The listing builds one solid part. Answer for the finished solid, in the listing's coordinates (mm). A direction names the side the tool comes from. Give positions to 0.01 mm unless a question says otherwise; leave off trailing zeros. Write each loop counter-clockwise with the first axis right and the second up, starting at its lowest first coordinate (ties: lowest second). Pieces come first, ordered by that corner, then holes. Notation, with made-up numbers: (-22.75, 39) - (20.25, 39) arc R16 ccw to (20.25, 54) - close; hole circle Ø11 at (32, 9). An arc over 180 degrees is marked (long way). Answer as CSV lines item,"result". Start each with the question number.
(1) Find section C-C (y = -13.5). Write down the section's boundary in (x, z).
(2) Straight lines are drawn through the part: probe 1 along X at (y, z) = (-4.5, 25); probe 2 along Z at (x, y) = (8.5, -11); probe 3 along Y at (x, z) = (-34, -5). For each, find the intervals that lie inside material, in ascending order.
(3) Each of these flat-tipped pins is pushed along its axis until it touches: pin 1 Ø12 at (x, y) = (2, -28.5) entering from -Z; pin 2 Ø9 at (y, z) = (-27.5, 2.5) entering from +X; pin 3 Ø9 at (x, y) = (-1.5, -30.5) entering from +Z. Where does it stop, or does it pass through?
(4) Find section B-B (z = 32). Write down the section's boundary in (x, y).
(5) Find section D-D (x = 18.5). Write down the section's boundary in (y, z), then the cut area to 3 significant figures.
(6) Find section A-A (x = -35). Write down the section's boundary in (y, z).
(7) For faces 1 (the face through (-7.337, -2.702, 23.943)), 2 (the face through (7.287, -33.942, 7.248)), 3 (the face through (-7.248, -33.942, -7.287)), 4 (the face through (8.05, -10, 24)), determine the directions among +Z, -Z, +X, -X, +Y, -Y from which every point of the face is accessible in a straight line to the end or side of a thin tool.
from build123d import *

# Parameters (mm, degrees)
F0_W     = 16
F0_H     = 16
F1_DEPTH = 50
F0_W_2   = 20
F0_H_2   = 20
F2_DEPTH = 20
F3_W     = 16
F3_H     = 16
F4_DEPTH = 40
F5_W     = 16
F5_H     = 16
F6_DEPTH = 40
F7_W     = 16.1
F7_H     = 16.1
F8_DEPTH = 40
F9_R     = 2.5


with BuildPart() as f1:
    # F0 (on Front) → F1 (new body)
    with BuildSketch(Plane.XZ):
        Rectangle(F0_W, F0_H)
    extrude(amount=F1_DEPTH)

    # F0 (on Front) → F2 (join)
    with BuildSketch(Plane.XZ):
        Rectangle(F0_W_2, F0_H_2)
        Rectangle(F0_W, F0_H, mode=Mode.SUBTRACT)
    extrude(amount=F2_DEPTH)

    # F3 (on Right) → F4 (join)
    with BuildSketch(Plane.YZ):
        with Locations((-9.85, 0)):
            Rectangle(F3_W, F3_H)
    extrude(amount=F4_DEPTH)

    # F5 (on Right) → F6 (join)
    with BuildSketch(Plane.YZ):
        with Locations((-10, 0)):
            Rectangle(F5_W, F5_H)
    extrude(amount=-F6_DEPTH)

    # F7 (on Top) → F8 (join)
    with BuildSketch(Plane.XY):
        with Locations((0, -10)):
            Rectangle(F7_W, F7_H)
    extrude(amount=F8_DEPTH)

    # F9
    f9_edges = [f1.edges().sort_by_distance(p)[0] for p in [
        (0, 0, -10),
        (-25, -2, -8),
        (-25, -18, -8),
        (-25, -2, 8),
        (-25, -18, 8),
        (-40, -10, -8),
        (-40, -2, 0),
        (-40, -10, 8),
        (-40, -18, 0),
        (-8.05, -18.05, 25),
        (0, -18.05, 40),
        (-8.05, -10, 40),
        (8.05, -10, 40),
        (0, -1.95, 40),
        (-8.05, -1.95, 25),
        (8.05, -1.95, 25),
        (8.05, -18.05, 25),
        (-8, -35, 8),
        (0, -50, 8),
        (8, -35, 8),
        (-8, -50, 0),
        (0, -50, -8),
        (8, -50, 0),
        (25, -17.85, 8),
        (25, -17.85, -8),
        (40, -9.85, -8),
        (40, -1.85, 0),
        (40, -9.85, 8),
        (40, -17.85, 0),
        (8, -35, -8),
        (-8, -35, -8),
        (25, -1.85, -8),
    ]]
    fillet(f9_edges, radius=F9_R)


solid = f1.part
Result set:
1,outline,"(-40, -5.5) arc R2.5 ccw to (-37.5, -8) - (-10, -8) - (-10, -10) - (10, -10) - (10, -8) - (37.5, -8) arc R2.5 ccw to (40, -5.5) - (40, 5.5) arc R2.5 ccw to (37.5, 8) - (10, 8) - (10, 10) - (8.05, 10) - (8.05, 37.5) arc R2.5 ccw to (5.55, 40) - (-5.55, 40) arc R2.5 ccw to (-8.05, 37.5) - (-8.05, 10) - (-10, 10) - (-10, 8) - (-37.5, 8) arc R2.5 ccw to (-40, 5.5) - close"
2,probe 1,"-8.05 to 8.05"
2,probe 2,"-10 to 10"
2,probe 3,"-18 to -2"
3,pin 1,"z = -8"
3,pin 2,"x = 8"
3,pin 3,"z = 8"
4,outline,"(-8.05, -15.55) arc R2.5 ccw to (-5.55, -18.05) - (5.55, -18.05) arc R2.5 ccw to (8.05, -15.55) - (8.05, -4.45) arc R2.5 ccw to (5.55, -1.95) - (-5.55, -1.95) arc R2.5 ccw to (-8.05, -4.45) - close"
5,outline,"(-17.85, -5.5) arc R2.5 ccw to (-15.35, -8) - (-4.35, -8) arc R2.5 ccw to (-1.85, -5.5) - (-1.85, 8) - (-15.35, 8) arc R2.5 ccw to (-17.85, 5.5) - close"
5,area,"252 mm^2"
6,outline,"(-18, -5.5) arc R2.5 ccw to (-15.5, -8) - (-4.5, -8) arc R2.5 ccw to (-2, -5.5) - (-2, 5.5) arc R2.5 ccw to (-4.5, 8) - (-15.5, 8) arc R2.5 ccw to (-18, 5.5) - close"
7,face 1,"+Z, -X, +Y"
7,face 2,"+Z, +X, -Y"
7,face 3,"-Z, -X, -Y"
7,face 4,"+Z, +X, +Y, -Y"
